```python
from build123d import *

# Parameters (mm, degrees)
F1_DEPTH = 152.4
F0_R     = 8.277939
F2_DEPTH = 25.4
F5_R     = 8.277939
F6_DEPTH = 25.4
F7_R     = 8.277939
F8_DEPTH = 25.4


with BuildPart() as f1:
    # F0 (on Top) → F1 (new body)
    with BuildSketch(Plane.XY):
        with BuildLine():
            ThreePointArc((-13.505174, -3.321212), (-13.907558, 0), (-13.505174, 3.321212))
            Line((-13.505174, 3.321212), (-58.726565, 3.321212))
            Line((-58.726565, 3.321212), (-58.726565, -3.321212))
            Line((-58.726565, -3.321212), (-13.505174, -3.321212))
        make_face()
    extrude(amount=F1_DEPTH)

    # F0 (on Top) → F2 (join)
    with BuildSketch(Plane.XY):
        with BuildLine():
            ThreePointArc((13.907558, 0), (1.672749, 13.806595), (-13.505174, 3.321212))
            ThreePointArc((-13.505174, 3.321212), (-13.907558, 0), (-13.505174, -3.321212))
            ThreePointArc((-13.505174, -3.321212), (1.672749, -13.806595), (13.907558, 0))
        make_face()
        Circle(F0_R, mode=Mode.SUBTRACT)
    extrude(amount=F2_DEPTH)

    # F5 (on offset) → F6 (join)
    with BuildSketch(Plane.XY.offset(50.8)):
        with BuildLine():
            ThreePointArc((-13.505174, -3.321212), (13.907558, 0), (-13.505174, 3.321212))
            ThreePointArc((-13.505174, 3.321212), (-13.907558, 0), (-13.505174, -3.321212))
        make_face()
        Circle(F5_R, mode=Mode.SUBTRACT)
    extrude(amount=F6_DEPTH)

    # F7 (on offset) → F8 (join)
    with BuildSketch(Plane.XY.offset(101.6)):
        with BuildLine():
            ThreePointArc((-13.505174, -3.321212), (13.907558, 0), (-13.505174, 3.321212))
            ThreePointArc((-13.505174, 3.321212), (-13.907558, 0), (-13.505174, -3.321212))
        make_face()
        Circle(F7_R, mode=Mode.SUBTRACT)
    extrude(amount=F8_DEPTH)


solid = f1.part
```
Here's how the part is built. I have some questions about the finished solid (model axes, mm). A direction names the side the tool comes from. Coordinates: 2 decimals unless noted, no trailing zeros. Write each loop counter-clockwise with the first axis right and the second up, starting at its lowest first coordinate (ties: lowest second). Pieces come first, ordered by that corner, then holes. Notation, with made-up numbers: (75, -38.5) -> (130, -38.5) arc R35 ccw to (130, -5.5) -> close; hole circle Ø5 at (17.5, -29). An arc over 180 degrees is marked (long way). Use a Markdown table: item, result. Add a question column.
(1) Please list where these lines run through material, in increasing order: line 1 (Z direction, x = 10.5, y = 0); line 2 (Y direction, x = 0, z = 19.75); line 3 (X direction, y = -0.5, z = 117.5).
(2) If we section it at D-D, the plane z = 81.5: Write out the boundary of the cut face in (x, y).
(3) We'd pull the mould along Y, two halves only. Please class faces 1 (the flat face through (-36, -3.321, 75)), 2 (the cylindrical face through (13.896, -0.565, 114.122)), 3 (the cylindrical face through (-1.794, -8.081, 114.122)), 4 (the flat face through (-36, 0, 152.4)): +Y half, -Y half, draft (parallel to the pull), parting line (faces both ways), or undercut.
(4) If we section it at C-C, the plane y = 6: Write out the boundary of the cut face in (x, z), and give its area (3 significant figures).
(5) If we section it at B-B, the plane z = 103.5: Write out the boundary of the cut face in (x, y).
(6) For faces 5 (the flat face through (-36, 3.321, 75)), 6 (the cylindrical face through (-13.907, -0.047, 37.922)), 7 (the cylindrical face through (-13.907, -0.047, 139.522)), which set-ups out of +Z, -Z, +X, -X, +Y, -Y let a thin tool reach every point of the face, with its end or its side?
(7) If we section it at A-A, the plane x = 0: Write out the boundary of the cut face in (y, z), and give its area (3 significant figures).
(8) I'm going to push flat-ended pins straight in: P1, Ø8.5, axis at x = -1.5, y = 1, coming from the +Z side; P2, Ø12, axis at x = -7, y = 2, coming from the +Z side; P3, Ø3, axis at y = -8, z = 124, coming from the -X side; P4, Ø8, axis at y = -11, z = 59, coming from the +X side. Where does each tip first touch, or does it pass through?
Outcome:
| question | item | result |
|---|---|---|
| 1 | line 1 | z = 0 to 25.4, 50.8 to 76.2, 101.6 to 127 |
| 1 | line 2 | y = -13.91 to -8.28, 8.28 to 13.91 |
| 1 | line 3 | x = -58.73 to -8.26, 8.26 to 13.9 |
| 2 | outline | (-58.73, -3.32) -> (-13.51, -3.32) arc R13.91 cw to (-13.51, 3.32) -> (-58.73, 3.32) -> close |
| 3 | face 1 | -Y half |
| 3 | face 2 | parting line |
| 3 | face 3 | undercut |
| 3 | face 4 | draft |
| 4 | outline | (-12.55, 0) -> (-5.7, 0) -> (-5.7, 25.4) -> (-12.55, 25.4) -> close; (-12.55, 50.8) -> (-5.7, 50.8) -> (-5.7, 76.2) -> (-12.55, 76.2) -> close; (-12.55, 101.6) -> (-5.7, 101.6) -> (-5.7, 127) -> (-12.55, 127) -> close; (5.7, 0) -> (12.55, 0) -> (12.55, 25.4) -> (5.7, 25.4) -> close; (5.7, 50.8) -> (12.55, 50.8) -> (12.55, 76.2) -> (5.7, 76.2) -> close; (5.7, 101.6) -> (12.55, 101.6) -> (12.55, 127) -> (5.7, 127) -> close |
| 4 | area | 1,040 mm^2 |
| 5 | outline | (-58.73, -3.32) -> (-13.51, -3.32) arc R13.91 ccw (long way) to (-13.51, 3.32) -> (-58.73, 3.32) -> close; hole circle Ø16.56 at (0, 0) |
| 6 | face 5 | +Z, -Z, -X, +Y |
| 6 | face 6 | +X |
| 6 | face 7 | +Z, +X |
| 7 | outline | (-13.91, 0) -> (-8.28, 0) -> (-8.28, 25.4) -> (-13.91, 25.4) -> close; (-13.91, 50.8) -> (-8.28, 50.8) -> (-8.28, 76.2) -> (-13.91, 76.2) -> close; (-13.91, 101.6) -> (-8.28, 101.6) -> (-8.28, 127) -> (-13.91, 127) -> close; (8.28, 0) -> (13.91, 0) -> (13.91, 25.4) -> (8.28, 25.4) -> close; (8.28, 50.8) -> (13.91, 50.8) -> (13.91, 76.2) -> (8.28, 76.2) -> close; (8.28, 101.6) -> (13.91, 101.6) -> (13.91, 127) -> (8.28, 127) -> close |
| 7 | area | 858 mm^2 |
| 8 | P1 | passes through |
| 8 | P2 | stops at z = 127 |
| 8 | P3 | stops at x = -12.3 |
| 8 | P4 | stops at x = 12.02 |
